Here's how the part is built. I have some questions about the finished solid (model axes, mm). A direction names the side the tool comes from. Give positions to 0.01 mm unless a question says otherwise; leave off trailing zeros. Order: outer loops, then holes, each group sorted by start corner. A loop starts at its lowest first (then second) coordinate and runs counter-clockwise, first axis right, second up.
Autodesk Inventor part; units mm, degrees
ref_plane "Work Plane2" through (18.3579, -55.5766, 10.6113) normal (1, 0, 0) x (0, 1, 0)
ref_plane "YZ Plane" through (0, 0, 0) normal (1, 0, 0) x (0, 1, 0)
ref_plane "XZ Plane" through (0, 0, 0) normal (0, 1, 0) x (-1, 0, 0)
ref_plane "Work Plane1" through (44.4579, -56.5766, -83.6387) normal (-1, 0, 0) x (0, 0, 1)
sketch "Sketch1" plane through (44.4579, -56.5766, -83.6387) normal (-1, 0, 0) x (0, 0, 1)
  line L0 (90.4615, 0) -> (90.4615, 14.375)
  line L1 (90.4615, 14.375) -> (94.9615, 14.375)
  arc A0 (94.9615, 14.375) -> (122.2885, 14.375) centre (108.625, 15.375) ccw
  line L2 (122.2885, 14.375) -> (127, 14.375)
  line L3 (127, 14.375) -> (127, 30.5)
  line L4 (52.8275, 30.5) -> (127, 30.5)
  line L5 (52.8275, 30.5) -> (52.8275, 10)
  line L6 (52.8275, 10) -> (59.8275, 10)
  line L7 (59.8275, 10) -> (59.8275, 0)
  line L8 (59.8275, 0) -> (90.4615, 0)
  line L9 (119.625, 13.875) -> (120.125, 13.875)
  line L10 (120.125, 13.875) -> (120.125, 16.875)
  line L11 (120.125, 16.875) -> (119.625, 16.875)
  line L12 (119.625, 16.875) -> (119.625, 13.875)
  line L13 (97.125, 16.875) -> (96.625, 16.875)
  line L14 (96.625, 16.875) -> (96.625, 13.875)
  line L15 (96.625, 13.875) -> (97.125, 13.875)
  line L16 (97.125, 13.875) -> (97.125, 16.875)
  circle A1 centre (108.625, 15.375) radius 5
  circle A2 centre (108.625, 15.375) radius 13.7
  line L17 (90.4615, 14.375) -> (127, 14.375)
  line L18 (127, 14.375) -> (127, 30.5)
  line L19 (127, 30.5) -> (90.4615, 30.5)
  line L20 (90.4615, 30.5) -> (90.4615, 14.375)
  line L21 (90.4615, 16.375) -> (127, 16.375)
  point P0 (83.6387, 56.5766)
  point P1 (94.9615, 16.375)
  point P2 (122.2885, 16.375)
  point P3 (127, 16.375)
  dimension "d0" = 2
ref_plane "Work Plane2" through (18.3579, -55.5766, 10.6113) normal (1, 0, 0) x (0, 1, 0)
extrude "Extrusion1" add sketch "Sketch1" along normal up to surface (26.1 mm away) contours L20 L4 L3 L21 A2
sketch "Sketch2" plane through (44.4579, -26.0766, 43.3613) normal (0, 1, 0) x (1, 0, 0)
  line L0 (-26.1, 0) -> (-26.1, 4.7115)
  line L1 (0, 0) -> (-26.1, 0)
  line L2 (0, 4.7115) -> (0, 0)
  line L3 (0, 4.7115) -> (-26.1, 4.7115)
  line L4 (-26.1, 32.0385) -> (-26.1, 36.5385)
  line L5 (0, 32.0385) -> (-26.1, 32.0385)
  line L6 (0, 36.5385) -> (0, 32.0385)
  line L7 (0, 36.5385) -> (-26.1, 36.5385)
  line L8 (-3, 34.3385) -> (-23.1, 34.3385)
  line L9 (-23.1, 34.3385) -> (-23.1, 2.2)
  line L10 (-23.1, 2.2) -> (-3, 2.2)
  line L11 (-3, 2.2) -> (-3, 34.3385)
  point P0 (-44.4579, 43.3613)
  dimension "d3" = 2.2
  dimension "d4" = 2.2
  dimension "d5" = 3
  dimension "d6" = 3
hole "Hole1" at (41.4579, -26.0766, 9.0229) at (41.4579, -26.0766, 41.1613) at (21.3579, -26.0766, 41.1613) at (21.3579, -26.0766, 9.0229) direction (0, -1, 0) diameter 3.6 end through all countersink diameter 6.5 countersink angle 90
sketch "Sketch3" plane through (44.4579, -40.2016, 6.8229) normal (0, 0, -1) x (-1, 0, 0)
  line L0 (0, 14.125) -> (0.6078, 14.125)
  line L1 (0, 14.125) -> (0, 0)
  line L2 (0, 0) -> (26.1, 0)
  line L3 (26.1, 14.125) -> (26.1, 0)
  line L4 (25.4922, 14.125) -> (26.1, 14.125)
  line L5 (5.3922, 14.125) -> (20.7078, 14.125)
  line L6 (12.3, 0.5) -> (12.3, -2.5)
  line L7 (12.3, 0.5) -> (6.3, 0.5)
  line L8 (6.3, -2.5) -> (6.3, 0.5)
  line L9 (12.3, -2.5) -> (6.3, -2.5)
  line L10 (12.3, -14.7) -> (12.3, 12.7)
  line L11 (26.1, -2) -> (26.1, -16.375)
  line L12 (23.1, -2) -> (26.1, -2)
  line L13 (3, -2) -> (23.1, -2)
  line L14 (0, -2) -> (3, -2)
  line L15 (0, -16.375) -> (0, -2)
  line L16 (0, -16.375) -> (26.1, -16.375)
  line L17 (12.3, -2) -> (5.3, -2)
  line L18 (5.3, -2) -> (5.3, 5)
  line L19 (5.3, 5) -> (12.3, 5)
  line L20 (12.3, 5) -> (12.3, -2)
  point P0 (44.4579, 40.2016)
  point P1 (12.3, 5)
  point P2 (5.3, -2)
  dimension "d14" = 7
  dimension "d15" = 7
extrude "Extrusion2" cut sketch "Sketch3" against normal blind 10 contours L18 L19 L10 L7 L8 L2 | L2 L8 L13 L18 | L8 L7 L6 L2 | L2 L6 L13 L8
properties part number "right_motor_ceil"
Q1. I need wall thicknesses on L1, parallel to X at y = -34.25, z = 9; L2, parallel to Z at x = 21.5, y = -29; L3, parallel to Z at x = 40, y = -35.5. Which ranges of each line are inside material? Lowest first, please.
Filled sheet:
L1: x = 18.36 to 19.56, 23.16 to 39.66, 43.26 to 44.46
L2: z = 6.82 to 7.23, 10.82 to 18.76, 31.22 to 39.37, 42.96 to 43.36
L3: z = 6.82 to 7.97, 10.08 to 12.53, 37.44 to 40.11, 42.22 to 43.36
Q2. For faces 5 (the face through (21.974, -27.275, 10.98)), 6 (the face through (32.158, -38, 9)), which set-ups out of +Z, -Z, +X, -X, +Y, -Y let a thin tool reach every point of the face, with its end or its side?
Filled sheet:
face 5: +Y
face 6: -Z, -Y
Q3. I'm going to push flat-ended pins straight in: P1, Ø4.5, axis at x = 21.36, z = 9.02, coming from the +Y side; P2, Ø3, axis at x = 41.46, z = 41.16, coming from the +Y side; P3, Ø6, axis at x = 41.46, z = 9.02, coming from the +Y side; P4, Ø1.8, axis at x = 37.5, z = 8.5, coming from the -Y side. Where does each tip first touch, or does it pass through?
Filled sheet:
P1: stops at y = -27.07
P2: passes through
P3: stops at y = -26.32
P4: stops at y = -35.2
Q4. If we section it at B-B on x = 27.25: List the corners of the cut face in (y, z) for me, plus the area to 3 significant figures.
Filled sheet:
outline: (-40.2, 6.82) - (-26.08, 6.82) - (-26.08, 43.36) - (-40.2, 43.36) - (-40.2, 38.65) arc R13.7 cw to (-40.2, 11.32) - close
area: 249 mm2
Q5. If we section it at C-C on y = -32.5: List the corners of the cut face in (x, z) for me.
Filled sheet:
outline: (18.36, 6.82) - (44.46, 6.82) - (44.46, 14.4) - (18.36, 14.4) - close; (18.36, 35.57) - (44.46, 35.57) - (44.46, 43.36) - (18.36, 43.36) - close; hole circle Ø3.6 at (21.36, 9.02); hole circle Ø3.6 at (21.36, 41.16); hole circle Ø3.6 at (41.46, 9.02); hole circle Ø3.6 at (41.46, 41.16)
Q6. If we section it at D-D on z = 25: List the corners of the cut face in (x, y) for me, plus the area to 3 significant figures.
Filled sheet:
outline: (18.36, -27.5) - (44.46, -27.5) - (44.46, -26.08) - (18.36, -26.08) - close
area: 37.2 mm2
Q7. If we section it at A-A on y = -29: List the corners of the cut face in (x, z) for me, plus the area to 3 significant figures.
Filled sheet:
outline: (18.36, 6.82) - (44.46, 6.82) - (44.46, 18.76) - (18.36, 18.76) - close; (18.36, 31.22) - (44.46, 31.22) - (44.46, 43.36) - (18.36, 43.36) - close; hole circle Ø3.6 at (21.36, 9.02); hole circle Ø3.6 at (21.36, 41.16); hole circle Ø3.6 at (41.46, 9.02); hole circle Ø3.6 at (41.46, 41.16)
area: 588 mm2
Q8. Thinking about a two-plate mould opening in Z: for faces 1 (the face through (31.591, -27.505, 24.699)), 2 (the face through (32, -33, 6.823)), 3 (the face through (32, -40.202, 41)), 4 (the face through (32, -33, 43.361)), which applies, released by +Z, released by -Z, zero draft, split by the parting line, or undercut?
Filled sheet:
face 1: undercut
face 2: released by -Z
face 3: zero draft
face 4: released by +Z
